Design review of the part shown in the three views and the two pictorial views. Dimensions are in mm from the part's minimum x, y and z. A direction names the side the tool comes from. Give positions to 0.01 mm unless a question says otherwise; leave off trailing zeros. Loops run counter-clockwise (first coordinate to the right, second up) from the corner with the lowest first, then second, coordinate; pieces in that order, holes last.
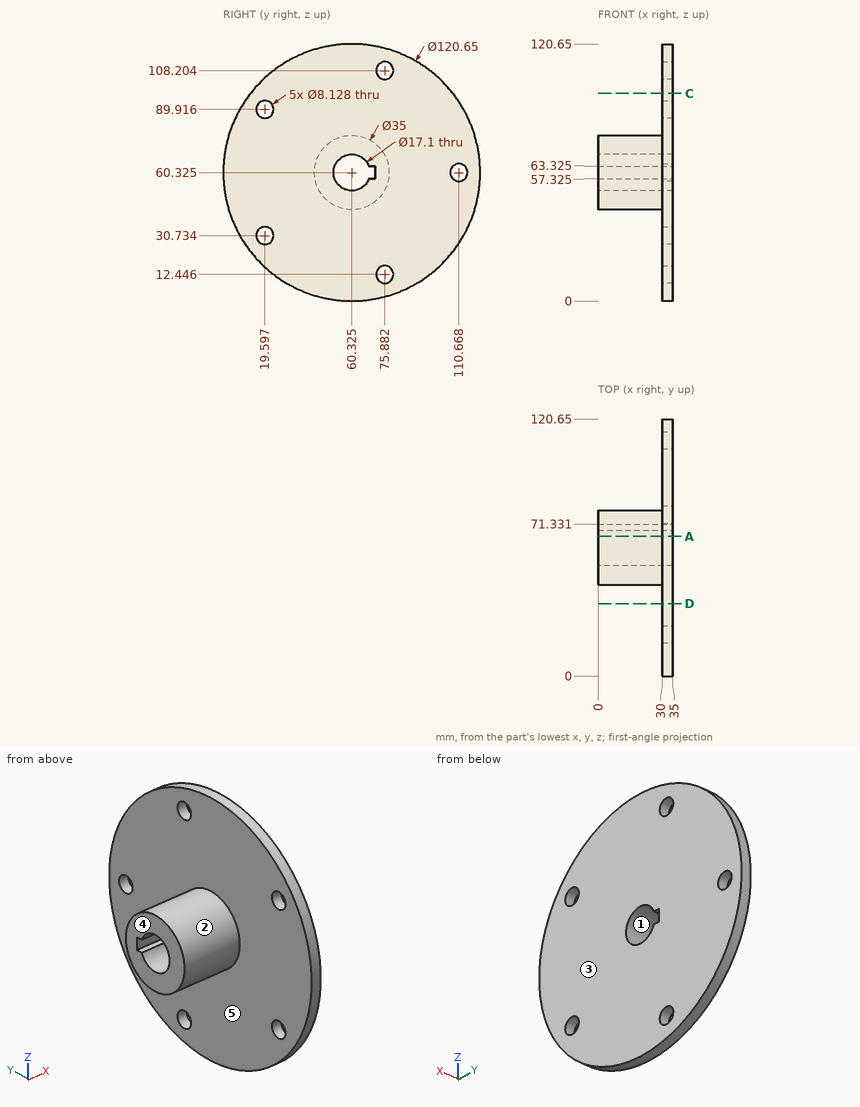
Q1. Consider section D-D on y = 34. Give the boundary of the cut face in (x, z), plus the area to 3 significant figures.
Answers:
outline: (30, 6.05) - (35, 6.05) - (35, 114.6) - (30, 114.6) - close
area: 543 mm2
Q2. Consider section C-C on z = 97.5. Give the boundary of the cut face in (x, y) (1 decimal), plus the area to 3 significant figures.
Answers:
outline: (30, 12.8) - (35, 12.8) - (35, 107.8) - (30, 107.8) - close
area: 475 mm2
Q3. Mouldability with a two-part tool opening along Z and no side actions: class the marked faces 1, 2 and 3 as +Z half, -Z half, draft (parallel to the pull), parting line (faces both ways), or undercut.
Answers:
face 1: undercut
face 2: parting line
face 3: draft
Q4. For pin 1 Ø5 at (y, z) = (19.6, 89.92) entering from -X; pin 2 Ø6.5 at (x, z) = (26, 61) entering from -Y (3 decimals); pin 3 Ø1.5 at (x, y) = (19.5, 69.5) entering from -Z; pin 4 Ø10.5 at (y, z) = (19.6, 30.73) entering from -X, all flat-tipped, find the tip position at first contact; note any pin that passes through.
Answers:
pin 1: passes through
pin 2: stops at y = 42.825
pin 3: stops at z = 44.99
pin 4: stops at x = 30
Q5. For probe 1 along Y at (x, z) = (18.5, 60.5); probe 2 along X at (y, z) = (26, 60.5); probe 3 along Z at (x, y) = (33.5, 43), list the stretches that pass through material, from the lowest coordinate up.
Answers:
probe 1: y = 42.83 to 51.78, 71.33 to 77.82
probe 2: x = 30 to 35
probe 3: z = 2.54 to 118.11
Q6. Machinability: for the marked faces 4 and 5, which of the approach directions +Z, -Z, +X, -X, +Y, -Y give a long, thin tool a straight path to every point of the face, cutting with its end or side? Answer none if there is none.
Answers:
face 4: +Z, -Z, -X, +Y, -Y
face 5: -X
Q7. Consider section A-A on y = 65.5. Give the boundary of the cut face in (x, z).
Answers:
outline: (0, 43.61) - (30, 43.61) - (30, 0.22) - (35, 0.22) - (35, 53.52) - (0, 53.52) - close; (0, 67.13) - (35, 67.13) - (35, 120.43) - (30, 120.43) - (30, 77.04) - (0, 77.04) - close
